from build123d import *

# Parameters (mm, degrees)
SKETCH095_W         = 108
SKETCH095_H         = 108
PAD041_DEPTH        = 100
SKETCH096_W         = 100
SKETCH096_H         = 100
POCKET036_DEPTH     = 98
FILLET002_R         = 8
SKETCH097_W         = 2
SKETCH097_H         = 92
SKETCH097_W_2       = 92
SKETCH097_H_2       = 2
POCKET037_DEPTH     = 98
REVOLUTION012_ANGLE = 180
POCKET038_DEPTH     = 2


with BuildPart() as part:
    # Sketch095 → Pad041 (new body)
    with BuildSketch(Plane.XY):
        with Locations((54, 54)):
            Rectangle(SKETCH095_W, SKETCH095_H)
    extrude(amount=PAD041_DEPTH)

    # Sketch096 (on Face6 of Pad041) → Pocket036 (cut)
    with BuildSketch(Plane.XY.offset(100)):
        with Locations((54, 54)):
            Rectangle(SKETCH096_W, SKETCH096_H)
    extrude(amount=-POCKET036_DEPTH, mode=Mode.SUBTRACT)

    # Fillet002
    fillet002_edges = [part.edges().sort_by_distance(p)[0] for p in [
        (108, 0, 50),
        (0, 0, 50),
        (0, 108, 50),
        (108, 108, 50),
    ]]
    fillet(fillet002_edges, radius=FILLET002_R)

    # Sketch097 (on Face5 of Fillet002) → Pocket037 (cut)
    with BuildSketch(Plane.XY.offset(100)):
        with Locations((3, 54)):
            Rectangle(SKETCH097_W, SKETCH097_H)
        with Locations((54, 3)):
            Rectangle(SKETCH097_W_2, SKETCH097_H_2)
        with Locations((105, 54)):
            Rectangle(SKETCH097_W, SKETCH097_H)
        with Locations((54, 105)):
            Rectangle(SKETCH097_W_2, SKETCH097_H_2)
    extrude(amount=-POCKET037_DEPTH, mode=Mode.SUBTRACT)

    # Sketch105 (on Face10 of Pocket037) → Revolution012 (revolve)
    with BuildSketch(Plane(origin=(0, 108, 0), x_dir=(-1, 0, 0), z_dir=(0, 1, 0))):
        Polygon((-75, 100), (-73, 100), (-54, 80), (-56, 80), align=None)
    revolve(axis=Axis((54, 108, 80), (0, 0, 1)), revolution_arc=REVOLUTION012_ANGLE)

    # Sketch106 (on Face12 of Revolution012) → Pocket038 (cut)
    with BuildSketch(Plane(origin=(0, 108, 0), x_dir=(-1, 0, 0), z_dir=(0, 1, 0))):
        Polygon((-73, 100), (-54, 80), (-35, 100), align=None)
    extrude(amount=-POCKET038_DEPTH, mode=Mode.SUBTRACT)


solid = part.part
Part model, mm, in its own coordinate system. A direction names the side the tool comes from. Give positions to 0.01 mm unless a question says otherwise; leave off trailing zeros. Loops run counter-clockwise (first coordinate to the right, second up) from the corner with the lowest first, then second, coordinate; pieces in that order, holes last. Notation, with made-up numbers: (-4, 69) -> (39, 69) arc R18 ccw to (39, 103) -> close; hole circle Ø1 at (30.5, -20). An arc over 180 degrees is marked (long way). Write each question's results on one line, items separated by ' | '. Start each with the question number.
Q1. Band-saw the part on A-A on z = 13.5. List the corners of the cut face in (x, y), plus the area to 3 significant figures.
Q2. Pull direction Y, two halves, no side cores. Call faces 1 (the face through (0, 53, 49)), 2 (the face through (53, 2, 52)), 3 (the face through (105.594, 2.281, 50.7)): +Y half, -Y half, draft (parallel to the pull), parting line (faces both ways), or undercut.
Q3. Pin check, flat tips, straight feed: P1, Ø5, axis at x = 54, y = 71.5, coming from the +Z side; P2, Ø2, axis at y = 102.5, z = 30.5, coming from the -X side; P3, Ø1, axis at x = 104.5, z = 49.5, coming from the +Y side; P4, Ø4.5, axis at x = 101, z = 75, coming from the -Y side. Stop position of each tip, or through.
Q4. Band-saw the part on D-D on y = 102. List the corners of the cut face in (x, z), plus the area to 3 significant figures.
Q5. Wall check: L1, parallel to Y at x = 26, z = 14.5; L2, parallel to Z at x = 99, y = 63. Give the ranges that are in metal, low to high.
Q6. Band-saw the part on B-B on y = 56. List the corners of the cut face in (x, z), plus the area to 3 significant figures.
Q7. Which spindle directions (+Z, -Z, +X, -X, +Y, -Y) get a long thin tool onto all of the face, cutting with end or side? Do faces 4 (the face through (63.633, 107.014, 90.14)), 5 (the face through (53, 55, 0)). Say none if no direction does.
Results are:
1) outline: (0, 8) arc R8 ccw to (8, 0) -> (100, 0) arc R8 ccw to (108, 8) -> (108, 100) arc R8 ccw to (100, 108) -> (8, 108) arc R8 ccw to (0, 100) -> close; hole (2, 8) -> (4, 8) -> (4, 4) -> (8, 4) -> (8, 2) -> (100, 2) -> (100, 4) -> (104, 4) -> (104, 8) -> (106, 8) -> (106, 100) -> (104, 100) -> (104, 104) -> (100, 104) -> (100, 106) -> (8, 106) -> (8, 104) -> (4, 104) -> (4, 100) -> (2, 100) -> close | area: 873 mm²
2) face 1: draft | face 2: undercut | face 3: -Y half
3) P1: stops at z = 2 | P2: stops at x = 0.14 | P3: stops at y = 106.93 | P4: stops at y = 0
4) outline: (0.25, 0) -> (107.75, 0) -> (107.75, 100) -> (104, 100) -> (104, 2) -> (4, 2) -> (4, 100) -> (0.25, 100) -> close | area: 949 mm²
5) L1: y = 0 to 2, 106 to 108 | L2: z = 0 to 2
6) outline: (0, 0) -> (108, 0) -> (108, 100) -> (106, 100) -> (106, 2) -> (2, 2) -> (2, 100) -> (0, 100) -> close | area: 608 mm²
7) face 4: +Z | face 5: -Z, +X, -X, +Y, -Y
